from build123d import *

# Parameters (mm, degrees)
CROQUIS1_R              = 18.4
SALIENTE_EXTRUIR1_DEPTH = 26.3
CORTAR_EXTRUIR1_START   = -5
CROQUIS2_R              = 1.25
CORTAR_EXTRUIR1_DEPTH   = 5
CROQUIS3_R              = 1.25
CORTAR_EXTRUIR2_DEPTH   = 5
CROQUIS7_R              = 18.4
CORTAR_EXTRUIR5_DEPTH   = 19.3
CROQUIS8_R              = 6
CORTAR_EXTRUIR6_DEPTH   = 1


with BuildPart() as part:
    # Croquis1 → Saliente-Extruir1 (new body)
    with BuildSketch(Plane.XY):
        Circle(CROQUIS1_R)
    extrude(amount=SALIENTE_EXTRUIR1_DEPTH)

    # Croquis2 → Cortar-Extruir1 (cut)
    with BuildSketch(Plane.XY.offset(26.3).offset(CORTAR_EXTRUIR1_START)):
        with Locations((0, 10)):
            Circle(CROQUIS2_R)
        with Locations((10, 0)):
            Circle(CROQUIS2_R)
        with Locations((0, -10)):
            Circle(CROQUIS2_R)
        with Locations((-10, 0)):
            Circle(CROQUIS2_R)
        with BuildLine():
            Line((-8.379185723, -12.62182641), (-12.62182641, -8.379185723))
            Line((-12.62182641, -8.379185723), (-14.957986577, -10.71534589))
            ThreePointArc((-14.957986577, -10.71534589), (-13.010764774, -13.010764774), (-10.71534589, -14.957986577))
            Line((-10.71534589, -14.957986577), (-8.379185723, -12.62182641))
        make_face()
    extrude(amount=CORTAR_EXTRUIR1_DEPTH, mode=Mode.SUBTRACT)

    # Croquis3 → Cortar-Extruir2 (cut)
    with BuildSketch(Plane(origin=(0, 0, 0), x_dir=(-1, 0, 0), z_dir=(0, 0, -1))):
        with Locations(Location((-10, 0, 0), (0, 0, 180))):
            Circle(CROQUIS3_R)
        with Locations(Location((0, 10, 0), (0, 0, 180))):
            Circle(CROQUIS3_R)
        with Locations(Location((10, 0, 0), (0, 0, 180))):
            Circle(CROQUIS3_R)
        with Locations(Location((0, -10, 0), (0, 0, 180))):
            Circle(CROQUIS3_R)
    extrude(amount=-CORTAR_EXTRUIR2_DEPTH, mode=Mode.SUBTRACT)

    # Croquis7 → Cortar-Extruir5 (cut)
    with BuildSketch(Plane(origin=(0, 0, 0), x_dir=(-1, 0, 0), z_dir=(0, 0, -1))):
        Circle(CROQUIS7_R)
    extrude(amount=-CORTAR_EXTRUIR5_DEPTH, mode=Mode.SUBTRACT)

    # Croquis8 → Cortar-Extruir6 (cut)
    with BuildSketch(Plane(origin=(0, 0, 19.3), x_dir=(-1, 0, 0), z_dir=(0, 0, -1))):
        Circle(CROQUIS8_R)
    extrude(amount=-CORTAR_EXTRUIR6_DEPTH, mode=Mode.SUBTRACT)


solid = part.part
Geometry: final body of the model. Coordinates: model frame, mm. A direction names the side the tool comes from. Give positions to 0.01 mm unless a question says otherwise; leave off trailing zeros. Write each loop counter-clockwise with the first axis right and the second up, starting at its lowest first coordinate (ties: lowest second). Pieces come first, ordered by that corner, then holes. Notation, with made-up numbers: (-11.5, 76) -> (34.5, 76) arc R24 cw to (34.5, 110) -> close; hole circle Ø4 at (72, -40). An arc over 180 degrees is marked (long way). Answer in a Markdown table with one row per item.
(1) Section query B-B on x = 0. Return loops of the section in (y, z), then the cut area to 3 significant figures.
Answers below:
| item | result |
|---|---|
| outline | (-18.4, 19.3) -> (-6, 19.3) -> (-6, 20.3) -> (6, 20.3) -> (6, 19.3) -> (18.4, 19.3) -> (18.4, 26.3) -> (11.25, 26.3) -> (11.25, 21.3) -> (8.75, 21.3) -> (8.75, 26.3) -> (-8.75, 26.3) -> (-8.75, 21.3) -> (-11.25, 21.3) -> (-11.25, 26.3) -> (-18.4, 26.3) -> close |
| area | 221 mm^2 |
(2) Draft query along X for faces 4 (the cylindrical face through (8.75, 0.05, 23.76)), 5 (the cylindrical face through (17.55, 5.53, 22.75)), 6 (the flat face through (4.35, 4.35, 19.3)). Return one class per face: +X half, -X half, draft (parallel to the pull), parting line (faces both ways), or undercut.
Answers below:
| item | result |
|---|---|
| face 4 | undercut |
| face 5 | parting line |
| face 6 | draft |
(3) Section query D-D on z = 20.75. Return loops of the section in (x, y).
Answers below:
| item | result |
|---|---|
| outline | circle Ø36.8 at (0, 0) |
(4) Ray query, line 1 along Y through (x, z) = (0, 23); line 2 along Y through (x, z) = (0, 19.75); line 3 along Y through (x, z) = (-11, 23). Return the intervals inside material, ascending. Write a range as [from, to].
Answers below:
| item | result |
|---|---|
| line 1 | [-18.4, -11.25], [-8.75, 8.75], [11.25, 18.4] |
| line 2 | [-18.4, -6], [6, 18.4] |
| line 3 | [-10, -0.75], [0.75, 14.75] |
(5) Pin query (flat end, axial travel): pin 1 (1.5 mm diameter, centred on y = 13, z = 21, fed in from +X); pin 2 (2 mm diameter, centred on x = 0, y = -10.5, fed in from +Z); pin 3 (3 mm diameter, centred on y = 11, z = 20.5, fed in from +X); pin 4 (2 mm diameter, centred on x = -12.5, y = -10, fed in from +Z). Return the tip coordinate at first contact, or that it passes through.
Answers below:
| item | result |
|---|---|
| pin 1 | x = 13.73 |
| pin 2 | z = 26.3 |
| pin 3 | x = 15.76 |
| pin 4 | z = 21.3 |
(6) Set-up query: faces 1 (the flat face through (-13.77, -9.53, 23.76)), 2 (the flat face through (0, 0, 20.3)), 3 (the flat face through (-10, -11, 24)). Return all of +Z, -Z, +X, -X, +Y, -Y with unobstructed straight access to the full face (end or side cutting, diameter ignored); none if empty.
Answers below:
| item | result |
|---|---|
| face 1 | +Z, -Y |
| face 2 | -Z |
| face 3 | +Z |
(7) Section query A-A on z = 24.75. Return loops of the section in (x, y), then the cut area to 3 significant figures.
Answers below:
| item | result |
|---|---|
| outline | (-14.96, -10.72) -> (-12.62, -8.38) -> (-8.38, -12.62) -> (-10.72, -14.96) arc R18.4 ccw (long way) to start; hole circle Ø2.5 at (-10, 0); hole circle Ø2.5 at (0, -10); hole circle Ø2.5 at (0, 10); hole circle Ø2.5 at (10, 0) |
| area | 1,020 mm^2 |
